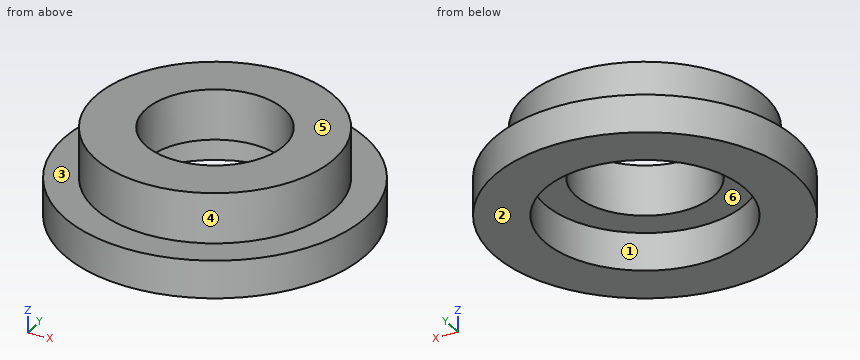
Autodesk Inventor part; units mm, degrees
ref_plane "YZ Plane" through (0, 0, 0) normal (1, 0, 0) x (0, 1, 0)
ref_plane "XZ Plane" through (0, 0, 0) normal (0, 1, 0) x (-1, 0, 0)
ref_plane "XY Plane" through (0, 0, 0) normal (0, 0, 1) x (1, 0, 0)
sketch "Sketch1" plane through (0, 0, 0) normal (0, 0, 1) x (1, 0, 0)
  circle A0 centre (0, 0) radius 2.75
  circle A1 centre (0, 0) radius 4.75
  dimension "d0" = 5.5
  dimension "d1" = 2
extrude "Extrusion1" add sketch "Sketch1" along normal blind 2
sketch "Sketch2" plane through (0, 0, 0) normal (0, 0, -1) x (-1, 0, 0)
  circle A0 centre (0, 0) radius 4.75
  circle A1 centre (0, 0) radius 4
  circle A2 centre (0, 0) radius 6
  dimension "d4" = 8
  dimension "d5" = 2
extrude "Extrusion2" add sketch "Sketch2" along normal blind 1.5 contours A0 | A2
properties part number "ArmBaseEncoderAlignmentFlange"
Here's how the part is built. I have some questions about the finished solid (model axes, mm). Face numbers are marked on the shaded views. A direction names the side the tool comes from. Coordinates: 2 decimals unless noted, no trailing zeros. Order: outer loops, then holes, each group sorted by start corner. A loop starts at its lowest first (then second) coordinate and runs counter-clockwise, first axis right, second up.
1) Will these pins go through, and if not, where does the flat tip stop? pin 1 (2 mm diameter, centred on x = 2.5, z = -0.5, fed in from +Y); pin 2 (2.5 mm diameter, centred on x = -2, y = 1.5, fed in from -Z); pin 3 (1.5 mm diameter, centred on y = 2.5, z = 1.5, fed in from +X).
2) Which directions (+Z, -Z, +X, -X, +Y, -Y) give clear straight access to the entire face, cutting with the end or side of a thin tool? Please do the marked faces 1, 2 and 3.
3) Imagine slicing it at A-A on x = 0. List the corners of the cut face in (y, z) for me, and give its area (3 significant figures).
4) We'd pull the mould along Z, two halves only. Please class the marked faces 4, 5 and 6: +Z half, -Z half, draft (parallel to the pull), parting line (faces both ways), or undercut.
5) Imagine slicing it at C-C on z = -0.9. List the corners of the cut face in (x, y) for me, and give its area (3 significant figures).
6) Imagine slicing it at D-D on x = 4.25. List the corners of the cut face in (y, z) for me.
7) I need wall thicknesses on line 1 (Y direction, x = 0, z = -0.9); line 2 (Y direction, x = 0, z = 1.5); line 3 (X direction, y = 0.5, z = -0.95). Which ranges of each line are inside material? Lowest first, please.
Response values:
1. pin 1: stops at y = 5.81
1. pin 2: stops at z = 0
1. pin 3: stops at x = 4.42
2. face 1: -Z
2. face 2: -Z, +X, -X, +Y, -Y
2. face 3: +Z
3. outline: (-6, -1.5) - (-4, -1.5) - (-4, 0) - (-2.75, 0) - (-2.75, 2) - (-4.75, 2) - (-4.75, 0) - (-6, 0) - close; (2.75, 0) - (4, 0) - (4, -1.5) - (6, -1.5) - (6, 0) - (4.75, 0) - (4.75, 2) - (2.75, 2) - close
3. area: 14.0 mm2
4. face 4: draft
4. face 5: +Z half
4. face 6: -Z half
5. outline: circle Ø12 at (0, 0); hole circle Ø8 at (0, 0)
5. area: 62.8 mm2
6. outline: (-4.24, -1.5) - (4.24, -1.5) - (4.24, 0) - (2.12, 0) - (2.12, 2) - (-2.12, 2) - (-2.12, 0) - (-4.24, 0) - close
7. line 1: y = -6 to -4, 4 to 6
7. line 2: y = -4.75 to -2.75, 2.75 to 4.75
7. line 3: x = -5.98 to -3.97, 3.97 to 5.98
